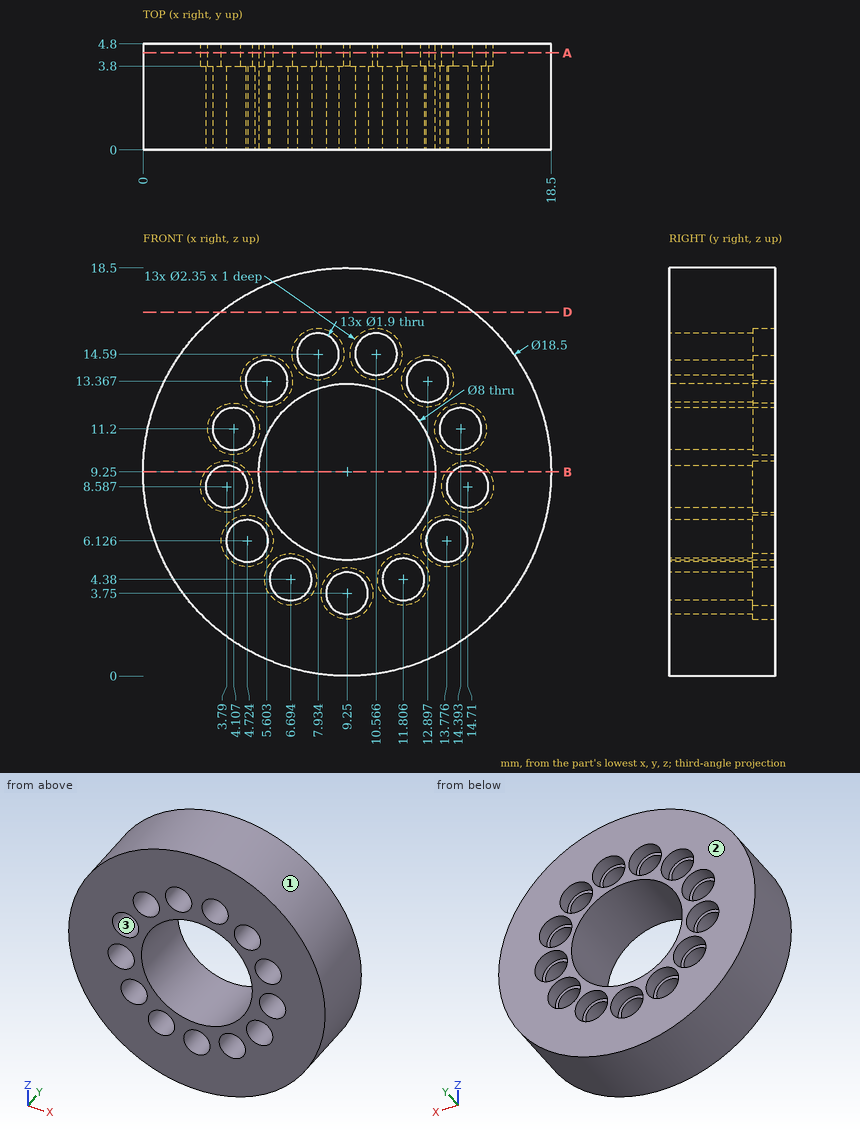
Check sheet for the drawn part. Datum: minimum x, y, z corner. Units: mm. Give positions to 0.01 mm unless a question says otherwise; leave off trailing zeros. Order: outer loops, then holes, each group sorted by start corner. A loop starts at its lowest first (then second) coordinate and runs counter-clockwise, first axis right, second up. Notation, with made-up numbers: (4, -24) -> (54, -24) arc R19 cw to (54, -8) -> close; hole circle Ø4 at (-3, -33.75). An arc over 180 degrees is marked (long way). One line per item, written item: value.
(1) Sectioned sample at D-D on z = 16.5. Record the cut outline in (x, y) (1 decimal).
Final values:
outline: (3.5, 0) -> (15, 0) -> (15, 4.8) -> (3.5, 4.8) -> close
(2) Draft check along Z on the marked faces 1, 2 and 3. Enter one of: pulls with the +Z half, pulls with the -Z half, needs draft (parallel to the pull), parting line crosses it, or undercut.
Final values:
face 1: parting line crosses it
face 2: needs draft
face 3: undercut
(3) Sectioned sample at B-B on z = 9.25. Record the cut outline in (x, y).
Final values:
outline: (0, 0) -> (3.11, 0) -> (3.11, 3.8) -> (2.82, 3.8) -> (2.82, 4.8) -> (0, 4.8) -> close; (4.47, 0) -> (5.25, 0) -> (5.25, 4.8) -> (4.76, 4.8) -> (4.76, 3.8) -> (4.47, 3.8) -> close; (13.25, 0) -> (14.03, 0) -> (14.03, 3.8) -> (13.74, 3.8) -> (13.74, 4.8) -> (13.25, 4.8) -> close; (15.39, 0) -> (18.5, 0) -> (18.5, 4.8) -> (15.68, 4.8) -> (15.68, 3.8) -> (15.39, 3.8) -> close
(4) Sectioned sample at A-A on y = 4.4. Count the separate pieces of the cut face and the enclosed holes in it, then the cut area to 3 significant figures.
Final values:
separate pieces: 1
enclosed holes: 14
area: 162 mm^2
(5) Scan lines: line 1 along Z through (x, y) = (9.25, 0.4); line 2 along Z through (x, y) = (14.5, 0.4) (1 decimal); line 3 along X through (y, z) = (0.25, 12.75) (1 decimal). Record each from-to range of solid material in increasing order. Write a range as [from, to].
Final values:
line 1: [0, 2.8], [4.7, 5.25], [13.25, 18.5]
line 2: [1.6, 5.5], [6.7, 7.7], [9.5, 10.3], [12.1, 16.9]
line 3: [0.7, 4.9], [6.3, 7.3], [11.2, 12.2], [13.6, 17.8]
(6) Gauge pin test, flat ends, axial feed: pin 1 (8 mm diameter, centred on x = 11, z = 2.5, fed in from -Y); pin 2 (1 mm diameter, centred on x = 11, y = 2, fed in from -Z) (1 decimal); pin 3 (2 mm diameter, centred on x = 7.93, z = 14.59, fed in from +Y); pin 4 (1.5 mm diameter, centred on x = 10.5, y = 1.5, fed in from -Z). Record the tip position at first contact, or that the pin passes through.
Final values:
pin 1: y = 0
pin 2: z = 0.1
pin 3: y = 3.8
pin 4: z = 0.01
